```python
from build123d import *

# Parameters (mm, degrees)
F0_W     = 30
F0_H     = 20
F1_DEPTH = 25
F2_R     = 7.5
F3_DEPTH = 26
F4_W     = 30
F4_H     = 25
F5_DEPTH = 3
F8_START = 25.6
F7_R     = 4
F8_DEPTH = 47.6
F9_START = 17.7
F6_R     = 2.5
F9_DEPTH = 70.5


with BuildPart() as f1:
    # F0 (on Front) → F1 (new body)
    with BuildSketch(Plane.XZ):
        with Locations((15, 10)):
            Rectangle(F0_W, F0_H)
    extrude(amount=F1_DEPTH)

    # F2 (on Top) → F3 (cut)
    with BuildSketch(Plane.XY):
        with Locations((14.9655956775, -11.9724776596)):
            Circle(F2_R)
    extrude(amount=F3_DEPTH, mode=Mode.SUBTRACT)

    # F4 (on Top) → F5 (join)
    with BuildSketch(Plane.XY):
        with Locations((15, -12.5)):
            Rectangle(F4_W, F4_H)
    extrude(amount=F5_DEPTH)

    # F7 (on Right) → F8 (join)
    with BuildSketch(Plane.YZ.offset(F8_START)):
        with Locations((-13.1077989936, 10.114679113)):
            Circle(F7_R)
    extrude(amount=F8_DEPTH)

    # F6 (on Right) → F9 (cut)
    with BuildSketch(Plane.YZ.offset(F9_START)):
        with Locations((-13.1077989936, 10.114679113)):
            Circle(F6_R)
    extrude(amount=F9_DEPTH, mode=Mode.SUBTRACT)


solid = f1.part
```
The model under review builds one solid part; all positions refer to its coordinate system, in mm. A direction names the side the tool comes from. Give positions to 0.01 mm unless a question says otherwise; leave off trailing zeros. Write each loop counter-clockwise with the first axis right and the second up, starting at its lowest first coordinate (ties: lowest second). Pieces come first, ordered by that corner, then holes.
(1) Consider section B-B, the plane z = 18.5. Give the boundary of the cut face in (x, y), and give its area (3 significant figures).
(2) Consider section D-D, the plane x = 61. Give the boundary of the cut face in (y, z).
(3) Consider section A-A, the plane y = -13.25. Give the boundary of the cut face in (x, z), and give its area (3 significant figures).
(4) Tool access review of faces 1 (the cylindrical face through (47.001, -15.605, 10.225)), 2 (the flat face through (15, -12, 0)): name each direction out of +Z, -Z, +X, -X, +Y, -Y from which nothing blocks a thin tool from reaching the whole face with its end or side.
(5) Consider section C-C, the plane x = 20. Give the boundary of the cut face in (y, z).
(6) For P1, Ø2, axis at x = 49, y = -18.5, coming from the +Z side; P2, Ø8, axis at x = 65, y = -18.5, coming from the -Z side; P3, Ø3, axis at y = -20.5, z = 5, coming from the +X side; P4, Ø4.5, axis at y = -13.11, z = 10.11, coming from the +X side, all flat-tipped, find the tip position at first contact; note any pin that passes through.
(7) The part is to be moulded in two halves that separate along Y. For faces 3 (the cylindrical face through (51.298, -17.104, 10.291)), 4 (the flat face through (73.2, -15, 8)), 5 (the flat face through (15, -12, 3)), 6 (the cylindrical face through (9.44, -6.9, 11.38)), say which applies: released by +Y, released by -Y, zero draft, split by the parting line, or undercut.
(8) To check wall thickness, follow L1, parallel to Y at x = 25.5, z = 10.25; L2, parallel to X at y = -10, z = 19; L3, parallel to Y at x = 17, z = 19.25. State the ranges of each line that lie inside material, in increasing order.
Returned:
1. outline: (0, -25) - (30, -25) - (30, 0) - (0, 0) - close; hole circle Ø15 at (14.97, -11.97)
1. area: 573 mm2
2. outline: circle Ø8 at (-13.11, 10.11); hole circle Ø5 at (-13.11, 10.11)
3. outline: (0, 0) - (30, 0) - (30, 6.12) - (73.2, 6.12) - (73.2, 7.62) - (22.36, 7.62) - (22.36, 3) - (7.58, 3) - (7.58, 20) - (0, 20) - close; (22.36, 12.61) - (73.2, 12.61) - (73.2, 14.11) - (30, 14.11) - (30, 20) - (22.36, 20) - close
3. area: 440 mm2
4. face 1: +X
4. face 2: -Z, +X, -X, +Y, -Y
5. outline: (-25, 0) - (0, 0) - (0, 20) - (-6.41, 20) - (-6.41, 3) - (-17.53, 3) - (-17.53, 20) - (-25, 20) - close
6. P1: passes through
6. P2: stops at z = 6.36
6. P3: stops at x = 30
6. P4: stops at x = 8.27
7. face 3: split by the parting line
7. face 4: zero draft
7. face 5: undercut
7. face 6: undercut
8. L1: y = -25 to -15.6, -10.61 to 0
8. L2: x = 0 to 7.73, 22.2 to 30
8. L3: y = -25 to -19.19, -4.75 to 0
